```python
from build123d import *

# Parameters (mm, degrees)
F0_W     = 50
F0_H     = 50
F1_DEPTH = 20
F2_R     = 2.828427
F3_DEPTH = 5
F4_R     = 1.5
F5_DEPTH = 25


with BuildPart() as f1:
    # F0 (on Top) → F1 (new body)
    with BuildSketch(Plane.XY):
        Rectangle(F0_W, F0_H)
    extrude(amount=F1_DEPTH)

    # F2 (on face) → F3 (cut)
    with BuildSketch(Plane.XY.offset(20)):
        Circle(F2_R)
    extrude(amount=-F3_DEPTH, mode=Mode.SUBTRACT)

    # F4 (on face) → F5 (cut)
    with BuildSketch(Plane.XY.offset(15)):
        Circle(F4_R)
    extrude(amount=-F5_DEPTH, mode=Mode.SUBTRACT)


solid = f1.part
```
CAD build for the part. Positions are in the model's coordinates, mm. A direction names the side the tool comes from. Round coordinates to 2 decimals unless told otherwise and drop trailing zeros. Loops run counter-clockwise (first coordinate to the right, second up) from the corner with the lowest first, then second, coordinate; pieces in that order, holes last. Notation, with made-up numbers: (41.25, 83.5) - (91.25, 83.5) arc R21 cw to (91.25, 111.5) - close; hole circle Ø6 at (10, 76.25). An arc over 180 degrees is marked (long way). Return JSON: item names as keys, results as strings. Group by question number.
Q1. Tool access for faces 4 (the face through (0, 6, 20)), 5 (the face through (-2.826, 0.124, 17.535)): list every direction of +Z, -Z, +X, -X, +Y, -Y with a clear straight run to the whole face (end or side of a thin tool).
Q2. Band-saw the part on A-A on y = 0. Give the cut face in (x, z), plus the area to 3 significant figures.
Q3. Drill centre lines: line 1 along Y through (x, z) = (0, 11.25); line 2 along Z through (x, y) = (-0.5, -2). Where is each one in solid material? Low to high. Write a range as [from, to].
Q4. Two-plate mould, pull along Y, no slides. Class faces 1 (the face through (0, -25, 10)), 2 (the face through (-25, 0, 10)), 3 (the face through (-1.5, 0.07, 7.6)): +Y half, -Y half, draft (parallel to the pull), parting line (faces both ways), or undercut.
Q5. Flat gauge pins, fed straight in: pin 1 Ø7.5 at (x, y) = (0, 0) entering from +Z; pin 2 Ø5 at (x, y) = (0, 0) entering from +Z. Where does each tip first touch, or does it go through?
Solutions:
{
 "1": {"face 4": "+Z, +X, -X, +Y, -Y", "face 5": "+Z"},
 "2": {"outline": "(-25, 0) - (-1.5, 0) - (-1.5, 15) - (-2.83, 15) - (-2.83, 20) - (-25, 20) - close; (1.5, 0) - (25, 0) - (25, 20) - (2.83, 20) - (2.83, 15) - (1.5, 15) - close", "area": "927 mm^2"},
 "3": {"line 1": "y = [-25, -1.5], [1.5, 25]", "line 2": "z = [0, 15]"},
 "4": {"face 1": "-Y half", "face 2": "draft", "face 3": "undercut"},
 "5": {"pin 1": "stops at z = 20", "pin 2": "stops at z = 15"}
}
